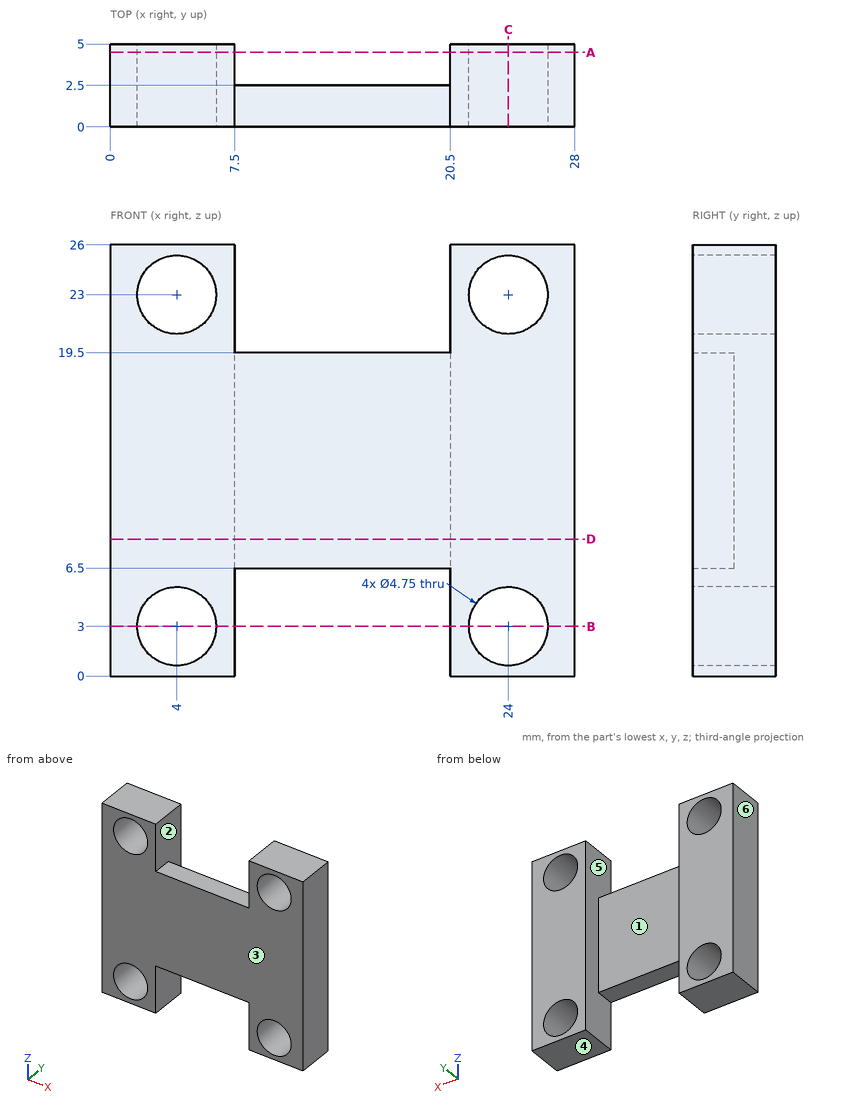
Job drawing, mm, ordinate dimensions from the low corner. One solid piece. A direction names the side the tool comes from. Give positions to 0.01 mm unless a question says otherwise; leave off trailing zeros. Order: outer loops, then holes, each group sorted by start corner. A loop starts at its lowest first (then second) coordinate and runs counter-clockwise, first axis right, second up. Notation, with made-up numbers: (17, -24) -> (55, -24) arc R19 ccw to (55, -19) -> close; hole circle Ø10 at (39, -22.75). An arc over 180 degrees is marked (long way). Return JSON: item names as keys, results as strings.
Q1. Saw through at C-C (x = 24). Write the cut outline in (y, z) (3 decimals).
Working result:
{"outline": "(0, 0) -> (5, 0) -> (5, 0.625) -> (0, 0.625) -> close; (0, 5.375) -> (5, 5.375) -> (5, 20.625) -> (0, 20.625) -> close; (0, 25.375) -> (5, 25.375) -> (5, 26) -> (0, 26) -> close"}
Q2. Saw through at A-A (y = 4.5). Write the cut outline in (x, z) (3 decimals).
Working result:
{"outline": "(0, 0) -> (7.5, 0) -> (7.5, 26) -> (0, 26) -> close; (20.5, 0) -> (28, 0) -> (28, 26) -> (20.5, 26) -> close; hole circle Ø4.75 at (4, 3); hole circle Ø4.75 at (4, 23); hole circle Ø4.75 at (24, 3); hole circle Ø4.75 at (24, 23)"}
Q3. Flat gauge pins, fed straight in: pin 1 (0.8 mm diameter, centred on x = 11, y = 1, fed in from -Z); pin 2 (3 mm diameter, centred on x = 16.5, y = 0.5, fed in from +Z); pin 3 (4.5 mm diameter, centred on x = 4, z = 23, fed in from -Y). Where does each tip first touch, or does it go through?
Working result:
{"pin 1": "z = 6.5", "pin 2": "z = 19.5", "pin 3": "through"}
Q4. Mould opens along X. For the marked faces 4, 5 and 6 say: pulls with the +X half, pulls with the -X half, needs draft (parallel to the pull), parting line crosses it, or undercut.
Working result:
{"face 4": "needs draft", "face 5": "undercut", "face 6": "pulls with the -X half"}
Q5. Drill centre lines: line 1 (Z direction, x = 4, y = 1.3) (3 decimals); line 2 (Z direction, x = 24.5, y = 1.4); line 3 (X direction, y = 3.6, z = 22). Where is each one in solid material? Low to high.
Working result:
{"line 1": "0 to 0.625, 5.375 to 20.625, 25.375 to 26", "line 2": "0 to 0.68, 5.32 to 20.68, 25.32 to 26", "line 3": "0 to 1.85, 6.15 to 7.5, 20.5 to 21.85, 26.15 to 28"}
Q6. Which spindle directions (+Z, -Z, +X, -X, +Y, -Y) get a long thin tool onto all of the face, cutting with end or side? Do the marked faces 1, 2 and 3. Say none if no direction does.
Working result:
{"face 1": "+Z, -Z, +Y", "face 2": "+Y", "face 3": "+Z, -Z, +X, -X, -Y"}
Q7. Saw through at B-B (z = 3). Write the cut outline in (x, y) (3 decimals), then the cut area to 3 significant figures.
Working result:
{"outline": "(0, 0) -> (1.625, 0) -> (1.625, 5) -> (0, 5) -> close; (6.375, 0) -> (7.5, 0) -> (7.5, 5) -> (6.375, 5) -> close; (20.5, 0) -> (21.625, 0) -> (21.625, 5) -> (20.5, 5) -> close; (26.375, 0) -> (28, 0) -> (28, 5) -> (26.375, 5) -> close", "area": "27.5 mm²"}
Q8. Saw through at D-D (z = 8.25). Write the cut outline in (x, y).
Working result:
{"outline": "(0, 0) -> (28, 0) -> (28, 5) -> (20.5, 5) -> (20.5, 2.5) -> (7.5, 2.5) -> (7.5, 5) -> (0, 5) -> close"}
